Could you check a few things on this drawing? It's one solid part, dimensions in mm from its lowest x, y, z. A direction names the side the tool comes from. Give positions to 0.01 mm unless a question says otherwise; leave off trailing zeros. Order: outer loops, then holes, each group sorted by start corner. A loop starts at its lowest first (then second) coordinate and runs counter-clockwise, first axis right, second up. Notation, with made-up numbers: (52, 9) - (64, 9) arc R11 ccw to (64, 23) - close; hole circle Ø4 at (-33, 81.25). An arc over 180 degrees is marked (long way). Return JSON: item names as keys, results as strings.
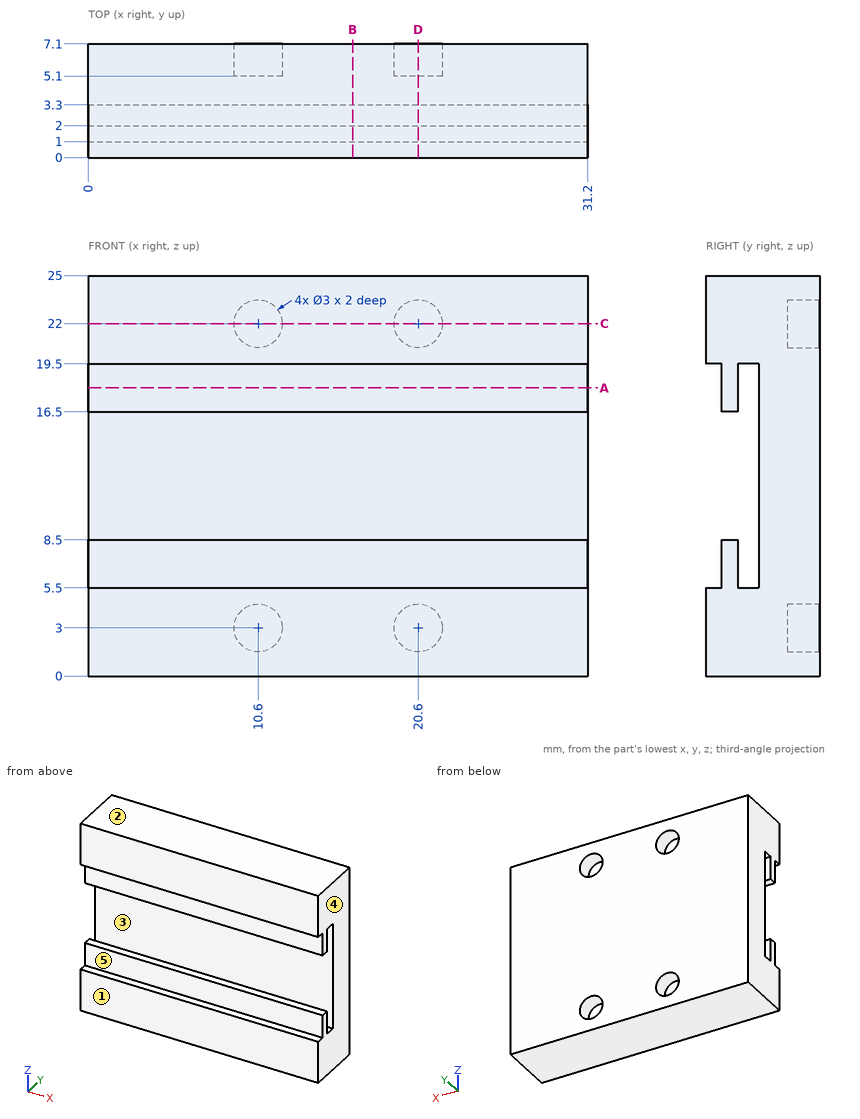
1. For pin 1 Ø0.9 at (x, z) = (20.5, 22.5) entering from +Y; pin 2 Ø2 at (x, z) = (20, 10) entering from -Y, each with a flat end and sliding along its axis, tell me the tip position at first contact or that it passes through.
Checks:
{"pin 1": "y = 5.1", "pin 2": "y = 3.3"}
2. Suppose I cut it at C-C (z = 22). List the corners of the cut face in (x, y) for me.
Checks:
{"outline": "(0, 0) - (31.2, 0) - (31.2, 7.1) - (22.1, 7.1) - (22.1, 5.1) - (19.1, 5.1) - (19.1, 7.1) - (12.1, 7.1) - (12.1, 5.1) - (9.1, 5.1) - (9.1, 7.1) - (0, 7.1) - close"}
3. Suppose I cut it at A-A (z = 18). List the corners of the cut face in (x, y) for me.
Checks:
{"outline": "(0, 1) - (31.2, 1) - (31.2, 2) - (0, 2) - close; (0, 3.3) - (31.2, 3.3) - (31.2, 7.1) - (0, 7.1) - close"}
4. Suppose I cut it at B-B (x = 16.5). List the corners of the cut face in (y, z) for me.
Checks:
{"outline": "(0, 0) - (7.1, 0) - (7.1, 25) - (0, 25) - (0, 19.5) - (1, 19.5) - (1, 16.5) - (2, 16.5) - (2, 19.5) - (3.3, 19.5) - (3.3, 5.5) - (2, 5.5) - (2, 8.5) - (1, 8.5) - (1, 5.5) - (0, 5.5) - close"}
5. Suppose I cut it at D-D (x = 20.6). List the corners of the cut face in (y, z) for me.
Checks:
{"outline": "(0, 0) - (7.1, 0) - (7.1, 1.5) - (5.1, 1.5) - (5.1, 4.5) - (7.1, 4.5) - (7.1, 20.5) - (5.1, 20.5) - (5.1, 23.5) - (7.1, 23.5) - (7.1, 25) - (0, 25) - (0, 19.5) - (1, 19.5) - (1, 16.5) - (2, 16.5) - (2, 19.5) - (3.3, 19.5) - (3.3, 5.5) - (2, 5.5) - (2, 8.5) - (1, 8.5) - (1, 5.5) - (0, 5.5) - close"}
6. If I drill on L1, parallel to X at y = 5.95, z = 22; L2, parallel to Z at x = 20.6, y = 5.95; L3, parallel to Z at x = 11, y = 2.5, over which ranges is the centre line in solid material (lowest first)? Write a range as [from, to].
Checks:
{"L1": "[0, 9.1], [12.1, 19.1], [22.1, 31.2]", "L2": "[0, 1.5], [4.5, 20.5], [23.5, 25]", "L3": "[0, 5.5], [19.5, 25]"}
7. Thinking about a two-plate mould opening in Y: for the marked faces 1, 2 and 3, which applies, +Y half, -Y half, draft (parallel to the pull), parting line (faces both ways), or undercut?
Checks:
{"face 1": "-Y half", "face 2": "draft", "face 3": "undercut"}
8. On a 3-axis mill with a long thin cutter (end or side, diameter ignored), from which of +Z, -Z, +X, -X, +Y, -Y can I reach the whole of each face in a straight line? I mean the marked faces 4 and 5. Say none if no direction works.
Checks:
{"face 4": "+Z, -Z, +X, +Y, -Y", "face 5": "+X, -X, -Y"}
